Geometry: final body of the model. Coordinates: model frame, mm. Round coordinates to 2 decimals unless told otherwise and drop trailing zeros. Loops run counter-clockwise (first coordinate to the right, second up) from the corner with the lowest first, then second, coordinate; pieces in that order, holes last. Notation, with made-up numbers: (75.5, 78) -> (89.5, 78) arc R25 cw to (89.5, 99) -> close; hole circle Ø8 at (-15, 80.5). An arc over 180 degrees is marked (long way). Answer in a Markdown table with one row per item.
```python
from build123d import *

# Parameters (mm, degrees)
F2_DEPTH = 170
F3_R     = 22.5
F4_DEPTH = 170
F6_DEPTH = 7


with BuildPart() as f2:
    # F1 (on face) → F2 (new body)
    with BuildSketch(Plane.XY):
        with BuildLine():
            ThreePointArc((27.4881675578, -0.8066252621), (27.4970417303, -0.4033560215), (27.5, 0))
            ThreePointArc((27.5, 0), (19.2877918034, 19.6018133689), (-0.4440790799, 27.4964141984))
            Line((-0.4440790799, 27.4964141984), (-0.4440790799, -0.5180921289))
            Line((-0.4440790799, -0.5180921289), (27.4881675578, -0.8066252621))
        make_face()
        with BuildLine():
            Line((-0.4440790799, -0.5180921289), (-0.4440790799, 27.4964141984))
            ThreePointArc((-0.4440790799, 27.4964141984), (-19.5732263839, -19.3168012084), (27.4881675578, -0.8066252621))
            Line((27.4881675578, -0.8066252621), (-0.4440790799, -0.5180921289))
        make_face()
    extrude(amount=F2_DEPTH)

    # F3 (on face) → F4 (cut)
    with BuildSketch(Plane.XY.offset(170)):
        Circle(F3_R)
    extrude(amount=-F4_DEPTH, mode=Mode.SUBTRACT)

    # F5 (on face) → F6 (cut)
    with BuildSketch(Plane(origin=(0, 0, 0), x_dir=(1, 0, 0), z_dir=(0, 0, -1))):
        with BuildLine():
            ThreePointArc((-5.5, 21.8174242293), (0, 22.5), (5.5, 21.8174242293))
            Line((5.5, 21.8174242293), (5.5, 26.9443871706))
            ThreePointArc((5.5, 26.9443871706), (2.7639964551, 27.3607442076), (0, 27.5))
            ThreePointArc((0, 27.5), (-2.7639964551, 27.3607442076), (-5.5, 26.9443871706))
            Line((-5.5, 26.9443871706), (-5.5, 21.8174242293))
        make_face()
    extrude(amount=-F6_DEPTH, mode=Mode.SUBTRACT)


solid = f2.part
```
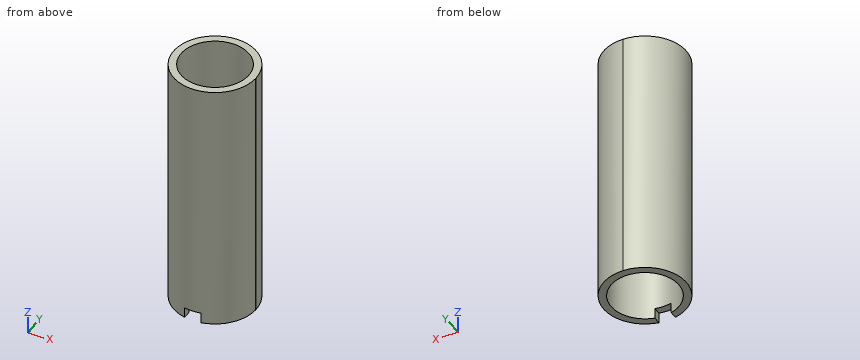
Item 1: Line query: probe 1 along X at (y, z) = (0, 109); probe 2 along Y at (x, z) = (-17, 152.5); probe 3 along Y at (x, z) = (-4.5, 53). Output: solid intervals per line, ascending. Write a range as [from, to].
Answer:
| item | result |
|---|---|
| probe 1 | x = [-27.5, -22.5], [22.5, 27.5] |
| probe 2 | y = [-21.62, -14.74], [14.74, 21.62] |
| probe 3 | y = [-27.13, -22.05], [22.05, 27.13] |
Item 2: Cut plane B-B (y = -15). Output: boundary loops of the cut face in (x, z).
Answer:
| item | result |
|---|---|
| outline | (-23.05, 0) -> (-16.77, 0) -> (-16.77, 170) -> (-23.05, 170) -> close; (16.77, 0) -> (23.05, 0) -> (23.05, 170) -> (16.77, 170) -> close |
Item 3: Cut plane C-C (z = 32). Output: boundary loops of the cut face in (x, y), then the cut area to 3 significant figures.
Answer:
| item | result |
|---|---|
| outline | circle Ø55 at (0, 0); hole circle Ø45 at (0, 0) |
| area | 785 mm² |
Item 4: Pin query (flat end, axial travel): pin 1 Ø4.5 at (x, y) = (-2, -25) entering from -Z; pin 2 Ø2 at (y, z) = (-5.5, 148.5) entering from +X; pin 3 Ø1 at (y, z) = (-21.5, 95) entering from -X. Return the tip coordinate at first contact, or that it passes through.
Answer:
| item | result |
|---|---|
| pin 1 | stops at z = 7 |
| pin 2 | stops at x = 27.13 |
| pin 3 | stops at x = -17.76 |
Item 5: Cut plane A-A (x = -13). Output: boundary loops of the cut face in (y, z), then the cut area to 3 significant figures.
Answer:
| item | result |
|---|---|
| outline | (-24.23, 0) -> (-18.36, 0) -> (-18.36, 170) -> (-24.23, 170) -> close; (18.36, 0) -> (24.23, 0) -> (24.23, 170) -> (18.36, 170) -> close |
| area | 2,000 mm² |
